Input: part model. Units: mm. Frame: model coordinates. Face numbers are marked on the shaded views. A direction names the side the tool comes from. Give positions to 0.01 mm unless a question says otherwise; leave off trailing zeros. Loops run counter-clockwise (first coordinate to the right, second up) from the corner with the lowest first, then second, coordinate; pieces in that order, holes last. Notation, with made-up numbers: (-25, 58) - (-21, 58) arc R8 cw to (-21, 66) - close; hole circle Ø11 at (12.5, 47). An arc over 180 degrees is marked (long way). Answer as a JSON object with one key per item and string values.
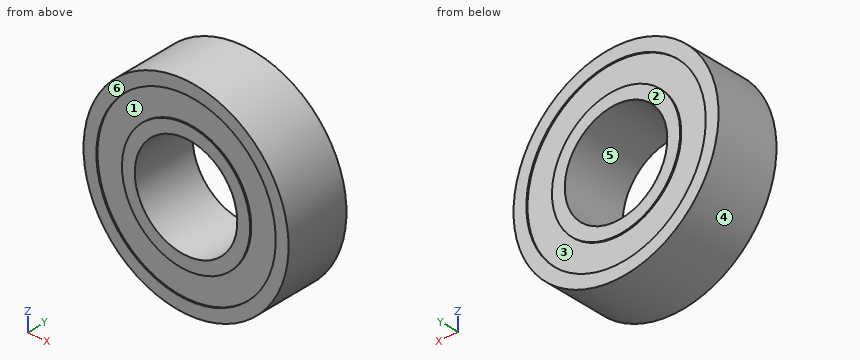
from build123d import *

# Parameters (mm, degrees)
SKETCH1_R      = 8
SKETCH1_R_2    = 4
EXTRUDE1_DEPTH = 5
SKETCH2_R      = 7
SKETCH2_R_2    = 5
EXTRUDE2_DEPTH = 0.1
EXTRUDE3_START = -0.1
SKETCH3_R      = 7
SKETCH3_R_2    = 5
EXTRUDE3_DEPTH = 0.1


with BuildPart() as part:
    # Sketch1 → Extrude1 (new body)
    with BuildSketch(Plane(origin=(0, 0, 0), x_dir=(1, 0, 0), z_dir=(0, 1, 0))):
        with Locations(Location((0, 0, 0), (0, 0, 270))):
            Circle(SKETCH1_R)
        with Locations(Location((0, 0, 0), (0, 0, 270))):
            Circle(SKETCH1_R_2, mode=Mode.SUBTRACT)
    extrude(amount=EXTRUDE1_DEPTH)

    # Sketch2 → Extrude2 (cut)
    with BuildSketch(Plane(origin=(0, 5, 0), x_dir=(1, 0, 0), z_dir=(0, 1, 0))):
        with Locations(Location((0, 0, 0), (0, 0, 270))):
            Circle(SKETCH2_R)
        with Locations(Location((0, 0, 0), (0, 0, 270))):
            Circle(SKETCH2_R_2, mode=Mode.SUBTRACT)
    extrude(amount=-EXTRUDE2_DEPTH, mode=Mode.SUBTRACT)

    # Sketch3 → Extrude3 (cut)
    with BuildSketch(Plane.XZ.offset(EXTRUDE3_START)):
        with Locations(Location((0, 0, 0), (0, 0, 90))):
            Circle(SKETCH3_R)
        with Locations(Location((0, 0, 0), (0, 0, 90))):
            Circle(SKETCH3_R_2, mode=Mode.SUBTRACT)
    extrude(amount=EXTRUDE3_DEPTH, mode=Mode.SUBTRACT)


solid = part.part
Item 1: Contact query for flat-ended pins moving along their axis: P1, Ø1.5, axis at x = 4.5, y = 0.5, coming from the -Z side; P2, Ø3, axis at y = 3.5, z = 2.5, coming from the -X side; P3, Ø1, axis at x = 5.5, y = 2, coming from the +Z side (3 decimals). Output: stop coordinate, or through.
Geometry check:
{"P1": "stops at z = -7.07", "P2": "stops at x = -7.94", "P3": "stops at z = 6.245"}
Item 2: Material intervals for line 1 (X direction, y = 4.95, z = 0); line 2 (X direction, y = 3.6, z = 0); line 3 (Y direction, x = 0.5, z = -6.75), sorted ascending. Write a range as [from, to].
Geometry check:
{"line 1": "x = [-8, -7], [-5, -4], [4, 5], [7, 8]", "line 2": "x = [-8, -4], [4, 8]", "line 3": "y = [0.1, 4.9]"}
Item 3: Cut plane D-D (y = 0.8). Return loops of the section in (x, z).
Geometry check:
{"outline": "circle Ø16 at (0, 0); hole circle Ø8 at (0, 0)"}
Item 4: Cut plane C-C (z = -6.75). Return loops of the section in (x, y), then the cut area to 3 significant figures.
Geometry check:
{"outline": "(-4.29, 0) - (-1.85, 0) - (-1.85, 0.1) - (1.85, 0.1) - (1.85, 0) - (4.29, 0) - (4.29, 5) - (1.85, 5) - (1.85, 4.9) - (-1.85, 4.9) - (-1.85, 5) - (-4.29, 5) - close", "area": "42.2 mm2"}
Item 5: Mould query, pull axis Z, two halves, no side actions, for the marked faces 4, 5 and 6. Classes: released by +Z, released by -Z, zero draft, split by the parting line, or undercut.
Geometry check:
{"face 4": "split by the parting line", "face 5": "undercut", "face 6": "zero draft"}
Item 6: Cut plane B-B (z = 0). Return loops of the section in (x, y), then the cut area to 3 significant figures.
Geometry check:
{"outline": "(-8, 0) - (-7, 0) - (-7, 0.1) - (-5, 0.1) - (-5, 0) - (-4, 0) - (-4, 5) - (-5, 5) - (-5, 4.9) - (-7, 4.9) - (-7, 5) - (-8, 5) - close; (4, 0) - (5, 0) - (5, 0.1) - (7, 0.1) - (7, 0) - (8, 0) - (8, 5) - (7, 5) - (7, 4.9) - (5, 4.9) - (5, 5) - (4, 5) - close", "area": "39.2 mm2"}
Item 7: Cut plane A-A (x = 0). Return loops of the section in (y, z).
Geometry check:
{"outline": "(0, -8) - (5, -8) - (5, -7) - (4.9, -7) - (4.9, -5) - (5, -5) - (5, -4) - (0, -4) - (0, -5) - (0.1, -5) - (0.1, -7) - (0, -7) - close; (0, 4) - (5, 4) - (5, 5) - (4.9, 5) - (4.9, 7) - (5, 7) - (5, 8) - (0, 8) - (0, 7) - (0.1, 7) - (0.1, 5) - (0, 5) - close"}
Item 8: Access query for the marked faces 1, 2 and 3. Directions: +Z, -Z, +X, -X, +Y, -Y. A direction counts if a zero-diameter tool reaches every point of the face in a straight line with its end or side. Return the directions, or none.
Geometry check:
{"face 1": "-Y", "face 2": "+Z, -Z, +X, -X, +Y", "face 3": "+Y"}
